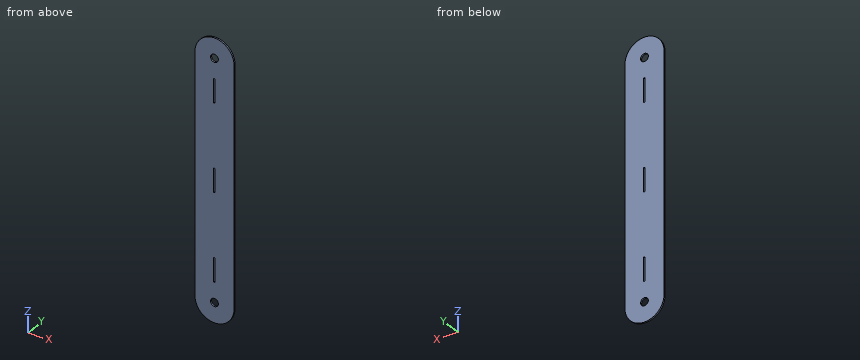
```python
from build123d import *

# Parameters (mm, degrees)
SKETCH1_R           = 2.5
SKETCH1_W           = 1
SKETCH1_H           = 15
BOSS_EXTRUDE1_DEPTH = 1


with BuildPart() as part:
    # Sketch1 → Boss-Extrude1 (new body)
    with BuildSketch(Plane(origin=(0, 0, 0), x_dir=(1, 0, 0), z_dir=(0, 1, 0))):
        with BuildLine():
            Line((12.5, 150), (12.5, 0))
            ThreePointArc((12.5, 0), (0, -12.5), (-12.5, 0))
            Line((-12.5, 0), (-12.5, 150))
            ThreePointArc((-12.5, 150), (0, 162.5), (12.5, 150))
        make_face()
        with Locations(Location((0, 0, 0), (0, 0, 270))):
            Circle(SKETCH1_R, mode=Mode.SUBTRACT)
        with Locations(Location((0, 150, 0), (0, 0, 270))):
            Circle(SKETCH1_R, mode=Mode.SUBTRACT)
        with Locations((0, 75)):
            Rectangle(SKETCH1_W, SKETCH1_H, mode=Mode.SUBTRACT)
        with Locations((0, 20)):
            Rectangle(SKETCH1_W, SKETCH1_H, mode=Mode.SUBTRACT)
        with Locations((0, 130)):
            Rectangle(SKETCH1_W, SKETCH1_H, mode=Mode.SUBTRACT)
    extrude(amount=BOSS_EXTRUDE1_DEPTH)


solid = part.part
```
Geometry check sheet. Reference: the model listing, model coordinates, mm. Round coordinates to 2 decimals unless told otherwise and drop trailing zeros. Loops run counter-clockwise (first coordinate to the right, second up) from the corner with the lowest first, then second, coordinate; pieces in that order, holes last. Notation, with made-up numbers: (81.5, 74) - (107.5, 74) arc R11 cw to (107.5, 89) - close; hole circle Ø6 at (44.25, -35). An arc over 180 degrees is marked (long way). Write item = value, one per line. Start each with the question number.
1. Section check A-A on y = 0.6. Enter the section's corners in (x, z).
2. Depth check by flat-ended pin: pin 1 (4 mm diameter, centred on x = 0, z = -150, fed in from -Y). Enter the tip coordinate at first touch or a pass-through.
3. Thickness scan on line 1 (X direction, y = 0.15, z = -14.5); line 2 (X direction, y = 0.5, z = -150); line 3 (Z direction, x = -3.5, y = 0.85). Record the ranges inside material, lowest first.
Working result:
q1.outline = (-12.5, -150) arc R12.5 ccw to (12.5, -150) - (12.5, 0) arc R12.5 ccw to (-12.5, 0) - close; hole circle Ø5 at (0, -150); hole circle Ø5 at (0, 0); hole (-0.5, -137.5) - (0.5, -137.5) - (0.5, -122.5) - (-0.5, -122.5) - close; hole (-0.5, -82.5) - (0.5, -82.5) - (0.5, -67.5) - (-0.5, -67.5) - close; hole (-0.5, -27.5) - (0.5, -27.5) - (0.5, -12.5) - (-0.5, -12.5) - close
q2.pin_1 = through
q3.line_1 = -12.5 to -0.5, 0.5 to 12.5
q3.line_2 = -12.5 to -2.5, 2.5 to 12.5
q3.line_3 = -162 to 12
